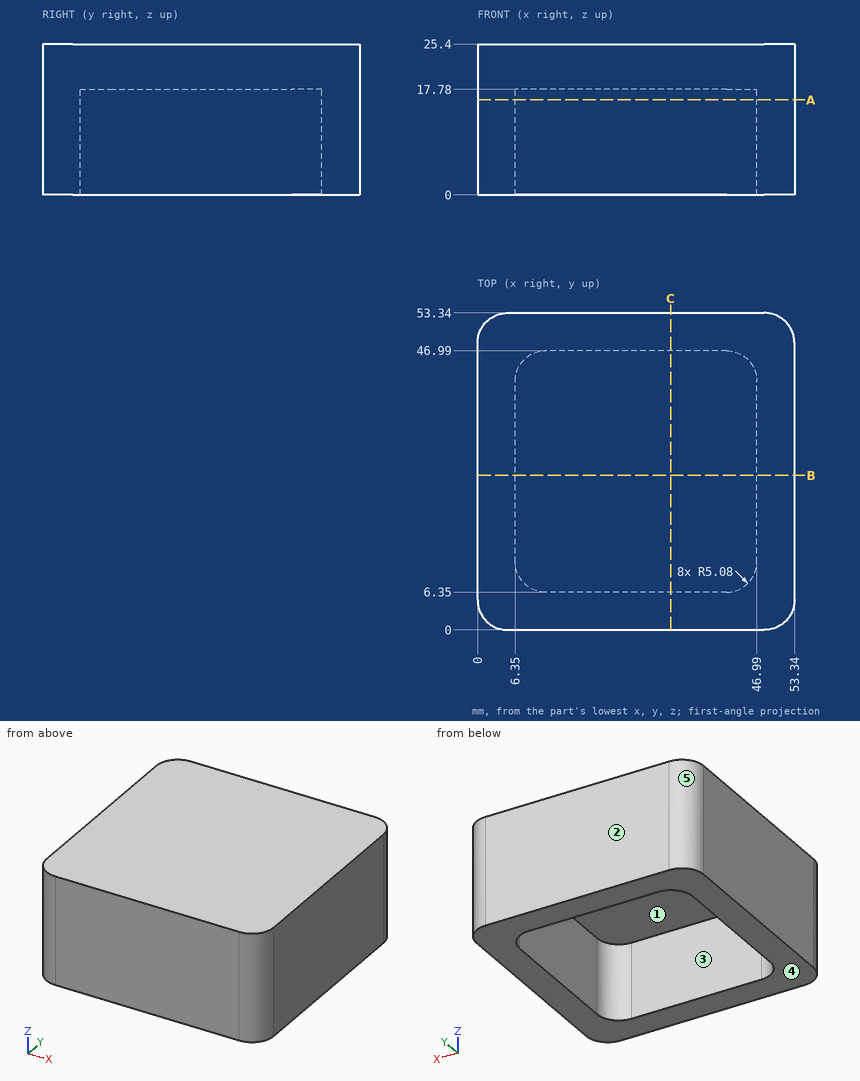
For this review, use the dimensioned drawing (mm, ordinates from the lowest corner) and the shaded views. A direction names the side the tool comes from. Give positions to 0.01 mm unless a question says otherwise; leave off trailing zeros. Loops run counter-clockwise (first coordinate to the right, second up) from the corner with the lowest first, then second, coordinate; pieces in that order, holes last.
Item 1: Tool access review of the marked faces 1 and 2: name each direction out of +Z, -Z, +X, -X, +Y, -Y from which nothing blocks a thin tool from reaching the whole face with its end or side.
Item 2: Draft analysis for pull direction Y (two halves, no side actions). For the marked faces 3, 4 and 5, state which applies: +Y half, -Y half, draft (parallel to the pull), parting line (faces both ways), or undercut.
Item 3: Take a section at A-A, the plane z = 16. State the section outline as (x, y) points.
Item 4: Insertion check: pin 1 (6 mm diameter, centred on x = 33, y = 29.5, fed in from -Z). The pin has a flat end and moves straight along its axis. Give the tip position at first contact, or say it passes through.
Item 5: Take a section at B-B, the plane y = 26. State the section outline as (x, z) points.
Item 6: For line 1 along X through (y, z) = (36, 2.5); line 2 along Z through (x, y) = (40, 18.5), list the stretches that pass through material, from the lowest coordinate up.
Calculated:
1. face 1: -Z
1. face 2: +Z, -Z, +X, -X, +Y
2. face 3: undercut
2. face 4: draft
2. face 5: +Y half
3. outline: (0, 5.08) arc R5.08 ccw to (5.08, 0) - (48.26, 0) arc R5.08 ccw to (53.34, 5.08) - (53.34, 48.26) arc R5.08 ccw to (48.26, 53.34) - (5.08, 53.34) arc R5.08 ccw to (0, 48.26) - close; hole (6.35, 11.43) arc R5.08 ccw to (11.43, 6.35) - (41.91, 6.35) arc R5.08 ccw to (46.99, 11.43) - (46.99, 41.91) arc R5.08 ccw to (41.91, 46.99) - (11.43, 46.99) arc R5.08 ccw to (6.35, 41.91) - close
4. pin 1: stops at z = 17.78
5. outline: (0, 0) - (6.35, 0) - (6.35, 17.78) - (46.99, 17.78) - (46.99, 0) - (53.34, 0) - (53.34, 25.4) - (0, 25.4) - close
6. line 1: x = 0 to 6.35, 46.99 to 53.34
6. line 2: z = 17.78 to 25.4
